Model file for the job. Use its own axes, mm. A direction names the side the tool comes from. Coordinates: 2 decimals unless noted, no trailing zeros. Order: outer loops, then holes, each group sorted by start corner. A loop starts at its lowest first (then second) coordinate and runs counter-clockwise, first axis right, second up. Notation, with made-up numbers: (38.25, -25.75) -> (77.25, -25.75) arc R17 cw to (77.25, -3.75) -> close; hole circle Ø1 at (35, 4). An arc over 180 degrees is marked (long way). Return JSON: item names as keys, results as strings. Group by question number.
1) Which spindle directions (+Z, -Z, +X, -X, +Y, -Y) get a long thin tool onto all of the face, cutting with end or side? Do faces 1 (the flat face through (8.21, -4.83, -3.57)), 2 (the cylindrical face through (-1.38, -6.2, 24.65)). Say none if no direction does.
2) Cut at A-A (z = 12). Write the cut outline in (x, y).
3) Flat gauge pins, fed straight in: pin 1 (10 mm diameter, centred on x = -4, z = 29, fed in from +Y); pin 2 (4 mm diameter, centred on x = 7.5, y = -6.5, fed in from +Z); pin 3 (2 mm diameter, centred on y = 0.5, z = 13.5, fed in from -X). Where does each tip first touch, or does it go through?
4) Probe line 1 (Z direction, x = -7, y = -1.5); line 2 (Z direction, x = -5.5, y = 2.5); line 3 (X direction, y = -2, z = 29). List the from-to ranges inside material, lowest first.
from build123d import *

# Parameters (mm, degrees)
HEAD_DEPTH         = 7.239
SKETCH2_R          = 6.35
SHAFT_DEPTH        = 50.8
SHAFT_CHAMFER_SIZE = 0.79375


with BuildPart() as part:
    # Head Sketch → Head (new body)
    with BuildSketch(Plane.XY):
        Polygon((10.998522628, 0), (5.499261314, 9.525), (-5.499261314, 9.525), (-10.998522628, 0), (-5.499261314, -9.525), (5.499261314, -9.525), align=None)
    extrude(amount=-HEAD_DEPTH)

    # Sketch9 → Head Chamfer (revolve, cut)
    with BuildSketch(Plane(origin=(0, 0, 0), x_dir=(1, 0, 0), z_dir=(0, 1, 0))):
        Polygon((10.998522628, 7.239), (9.525, 7.239), (10.998522628, 6.388261314), align=None)
    revolve(axis=Axis((0, 0, -10.14095), (0, 0, 1)), mode=Mode.SUBTRACT)

    # Sketch2 → Shaft (add)
    with BuildSketch(Plane.XY):
        Circle(SKETCH2_R)
    extrude(amount=SHAFT_DEPTH)

    # Shaft Chamfer
    shaft_chamfer_edges = [part.edges().sort_by_distance(p)[0] for p in [
        (-6.35, 0, 50.8),
    ]]
    chamfer(shaft_chamfer_edges, length=SHAFT_CHAMFER_SIZE)


solid = part.part
Answers below:
{
 "1": {"face 1": "+Z, -Z, +X, -Y", "face 2": "+Z"},
 "2": {"outline": "circle Ø12.7 at (0, 0)"},
 "3": {"pin 1": "stops at y = 6.35", "pin 2": "stops at z = 0", "pin 3": "stops at x = -6.35"},
 "4": {"line 1": "z = -7.24 to 0", "line 2": "z = -7.24 to 50.31", "line 3": "x = -6.03 to 6.03"}
}
